Build history of the part. All positions in model axes, mm. Face numbers are marked on the shaded views. A direction names the side the tool comes from. Give positions to 0.01 mm unless a question says otherwise; leave off trailing zeros. Write each loop counter-clockwise with the first axis right and the second up, starting at its lowest first coordinate (ties: lowest second). Pieces come first, ordered by that corner, then holes. Notation, with made-up numbers: (26, -22.5) -> (31, -22.5) arc R18 cw to (31, -18.5) -> close; hole circle Ø5 at (-10, 47). An arc over 180 degrees is marked (long way). Write item = value, one per line. Start each with the question number.
Q1. Saw through at D-D, the plane y = -55.5. List the corners of the cut face in (x, z), then the cut area to 3 significant figures.
Q2. Mould opens along X. For the marked faces 3, 4 and 5 say: pulls with the +X half, pulls with the -X half, needs draft (parallel to the pull), parting line crosses it, or undercut.
Q3. Saw through at B-B, the plane y = -38.1. List the corners of the cut face in (x, z), then the cut area to 3 significant figures.
Q4. Drop a flat-ended pin along its axis: P1, Ø10, axis at y = -38.1, z = 41.656, coming from the +X side. Give the stop position or say it passes through.
Q5. Tool access for the marked faces 1 and 2: list every direction of +Z, -Z, +X, -X, +Y, -Y with a clear straight run to the whole face (end or side of a thin tool).
Q6. Wall check: line 1 (X direction, y = -33.5, z = 50.5); line 2 (Z direction, x = -43.75, y = -38.1); line 3 (Z direction, x = 94.5, y = -51.5). Give the ranges that are in metal, low to high.
Q7. Saw through at A-A, the plane z = 12.5. List the corners of the cut face in (x, y).
Q8. Saw through at C-C, the plane z = 46. List the corners of the cut face in (x, y).
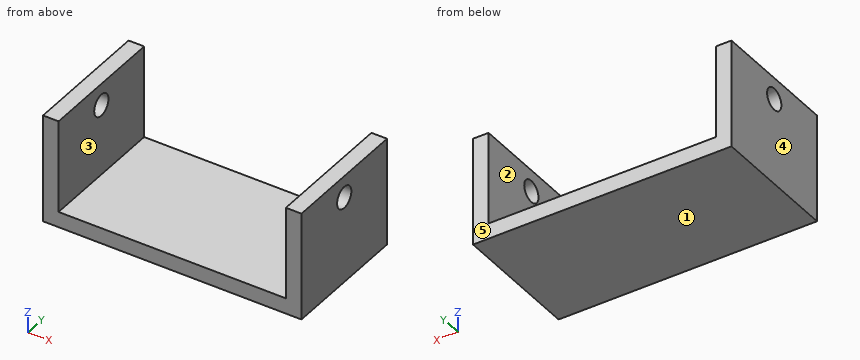
from build123d import *

# Parameters (mm, degrees)
F1_DEPTH = 76.2
F2_R     = 6.35
F3_DEPTH = 151.639


with BuildPart() as f1:
    # F0 (on Front) → F1 (new body)
    with BuildSketch(Plane.XZ):
        Polygon((94.677072, 0), (-38.672928, 0), (-38.672928, 54.356), (-47.816928, 54.356), (-47.816928, -9.144), (103.821072, -9.144), (103.821072, 54.356), (94.677072, 54.356), align=None)
    extrude(amount=F1_DEPTH)

    # F2 (on face) → F3 (cut, through all)
    with BuildSketch(Plane.YZ.offset(103.821072)):
        with Locations((-38.1, 41.656)):
            Circle(F2_R)
    extrude(amount=-F3_DEPTH, mode=Mode.SUBTRACT)


solid = f1.part
Report:
q1.outline = (-47.82, -9.14) -> (103.82, -9.14) -> (103.82, 54.36) -> (94.68, 54.36) -> (94.68, 0) -> (-38.67, 0) -> (-38.67, 54.36) -> (-47.82, 54.36) -> close
q1.area = 2,380 mm2
q2.face_3 = undercut
q2.face_4 = pulls with the -X half
q2.face_5 = needs draft
q3.outline = (-47.82, -9.14) -> (103.82, -9.14) -> (103.82, 35.31) -> (94.68, 35.31) -> (94.68, 0) -> (-38.67, 0) -> (-38.67, 35.31) -> (-47.82, 35.31) -> close; (-47.82, 48.01) -> (-38.67, 48.01) -> (-38.67, 54.36) -> (-47.82, 54.36) -> close; (94.68, 48.01) -> (103.82, 48.01) -> (103.82, 54.36) -> (94.68, 54.36) -> close
q3.area = 2,150 mm2
q4.P1 = through
q5.face_1 = -Z, +X, -X, +Y, -Y
q5.face_2 = +Z, +Y, -Y
q6.line_1 = -47.82 to -38.67, 94.68 to 103.82
q6.line_2 = -9.14 to 35.31, 48.01 to 54.36
q6.line_3 = -9.14 to 0
q7.outline = (-47.82, -76.2) -> (-38.67, -76.2) -> (-38.67, 0) -> (-47.82, 0) -> close; (94.68, -76.2) -> (103.82, -76.2) -> (103.82, 0) -> (94.68, 0) -> close
q8.outline = (-47.82, -76.2) -> (-38.67, -76.2) -> (-38.67, -42.73) -> (-47.82, -42.73) -> close; (-47.82, -33.47) -> (-38.67, -33.47) -> (-38.67, 0) -> (-47.82, 0) -> close; (94.68, -76.2) -> (103.82, -76.2) -> (103.82, -42.73) -> (94.68, -42.73) -> close; (94.68, -33.47) -> (103.82, -33.47) -> (103.82, 0) -> (94.68, 0) -> close
